from build123d import *

# Parameters (mm, degrees)
BOSS_EXTRUDE1_DEPTH = 3
CHAMFER1_SIZE       = 0.5


with BuildPart() as part:
    # Sketch1 → Boss-Extrude1 (new body)
    with BuildSketch(Plane.XZ):
        Polygon((-2.020725942, 3.5), (-4.041451884, 0), (-2.020725942, -3.5), (2.020725942, -3.5), (4.041451884, 0), (2.020725942, 3.5), align=None)
    extrude(amount=-BOSS_EXTRUDE1_DEPTH)

    # Sketch2 → Revolve1 (revolve)
    with BuildSketch(Plane(origin=(0, 0, 0), x_dir=(-1, 0, 0), z_dir=(0, 0, -1))):
        Polygon((-2.5, 3), (0, 3), (0, 10.5), (-3, 10.5), (-3, 4.5), (-2.5, 4.5), align=None)
    revolve(axis=Axis((0, 3, 0), (0, 1, 0)))

    # Sketch3 → Revolve2 (revolve)
    with BuildSketch(Plane.XY):
        Polygon((2.5, 0), (0, 0), (0, -2), (0.5, -2), align=None)
    revolve(axis=Axis((0, 0, 0), (0, -1, 0)))

    # Sketch4 → Cut-Revolve1 (revolve, cut)
    with BuildSketch(Plane(origin=(0, 0, 0), x_dir=(-1, 0, 0), z_dir=(0, 0, -1))):
        Polygon((-0.3, -2), (0, -2), (0, 10.5), (-1, 10.5), (-1, 0), (-0.75, -0.227272727), (-0.75, -0.7), (-0.3, -1.2), align=None)
    revolve(axis=Axis((0, -2, 0), (0, 1, 0)), mode=Mode.SUBTRACT)

    # Chamfer1
    chamfer1_edges = [part.edges().sort_by_distance(p)[0] for p in [
        (-3, 10.5, 0),
        (-1, 10.5, 0),
    ]]
    chamfer(chamfer1_edges, length=CHAMFER1_SIZE)


solid = part.part
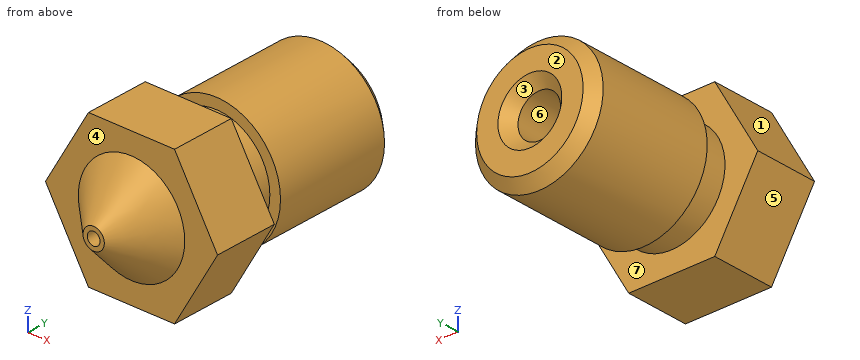
CAD build for the part. Positions are in the model's coordinates, mm. Face numbers are marked on the shaded views. A direction names the side the tool comes from. Round coordinates to 2 decimals unless told otherwise and drop trailing zeros. Order: outer loops, then holes, each group sorted by start corner. A loop starts at its lowest first (then second) coordinate and runs counter-clockwise, first axis right, second up. Notation, with made-up numbers: (68, 84) -> (93, 84) arc R27 ccw to (93, 108) -> close; hole circle Ø6 at (57.5, 61). An arc over 180 degrees is marked (long way). Write each question's results on one line, items separated by ' | '.
1. Wall check: line 1 along X through (y, z) = (-1.5, 0); line 2 along X through (y, z) = (5.5, 0). Give the ranges that are in metal, low to high. Write a range as [from, to].
Findings below:
line 1: x = [-1, -0.3], [0.3, 1] | line 2: x = [-3, -1], [1, 3]
2. Cut at B-B (y = 4). Give the cut face in (x, z), plus the area to 3 significant figures.
Findings below:
outline: circle Ø5 at (0, 0); hole circle Ø2 at (0, 0) | area: 16.5 mm²
3. Pull direction X, two halves, no side cores. Call the marked faces 1, 2 and 3: pulls with the +X half, pulls with the -X half, needs draft (parallel to the pull), parting line crosses it, or undercut.
Findings below:
face 1: pulls with the -X half | face 2: needs draft | face 3: undercut
4. Flat gauge pins, fed straight in: P1, Ø3.5, axis at x = 0, z = 0.5, coming from the +Y side; P2, Ø2, axis at y = 8, z = 1.5, coming from the -X side; P3, Ø1.5, axis at x = -1.5, y = 5, coming from the +Z side; P4, Ø1.5, axis at y = 7, z = -2, coming from the -X side. Where does each tip first touch, or does it go through?
Findings below:
P1: stops at y = 10.5 | P2: stops at x = -2.96 | P3: stops at z = 2.9 | P4: stops at x = -2.73
5. 3-axis set-ups, long thin cutter, end or side, ignore diameter. For the marked faces 4, 5, 6 and 7: which of +Z, -Z, +X, -X, +Y, -Y reach the whole face in a straight line?
Findings below:
face 4: -Y | face 5: -Z, -X, +Y, -Y | face 6: +Y | face 7: none
6. Cut at D-D (y = 7). Give the cut face in (x, z), plus the area to 3 significant figures.
Findings below:
outline: circle Ø6 at (0, 0); hole circle Ø2 at (0, 0) | area: 25.1 mm²
7. Cut at C-C (x = 3.25). Give the cut face in (y, z), plus the area to 4 significant figures.
Findings below:
outline: (0, -1.37) -> (3, -1.37) -> (3, 1.37) -> (0, 1.37) -> close | area: 8.225 mm²
